```python
from build123d import *

# Parameters (mm, degrees)
BASE_FLANGE1_DEPTH             = 400
SKETCH6_R                      = 2.5
CUT_EXTRUDE2_DEPTH             = 451
SKETCH10_R                     = 6
CUT_EXTRUDE1_DEPTH             = 451
KENAR_FLAN_1_STRIP_CUT_DEPTH   = 192.5268
KENAR_FLAN_1_STRIP_CUT_2_DEPTH = 192.5268
KENAR_FLAN_1_DEPTH             = 192.5268
KENAR_FLAN_1_BEND_DEPTH        = 192.5268


# Sheet-metal steps are written as plain solids
with BuildPart() as part:
    # Sketch1 → Base-Flange1 (new, symmetric)
    with BuildSketch(Plane(origin=(0, 0, 0), x_dir=(0, 0, -1), z_dir=(1, 0, 0))):
        with BuildLine():
            Line((-100, -50), (-100, -3.7366))
            ThreePointArc((-100, -3.7366), (-98.905575199, -1.094424801), (-96.2634, 0))
            Line((-96.2634, 0), (96.2634, 0))
            ThreePointArc((96.2634, 0), (98.905575199, -1.094424801), (100, -3.7366))
            Line((100, -3.7366), (100, -50))
            Line((100, -50), (97, -50))
            Line((97, -50), (97, -3.7366))
            ThreePointArc((97, -3.7366), (96.784254855, -3.215745145), (96.2634, -3))
            Line((96.2634, -3), (-96.2634, -3))
            ThreePointArc((-96.2634, -3), (-96.784254855, -3.215745145), (-97, -3.7366))
            Line((-97, -3.7366), (-97, -50))
            Line((-97, -50), (-100, -50))
        make_face()
    extrude(amount=BASE_FLANGE1_DEPTH, both=True)

    # Sketch6 → Cut-Extrude2 (cut, through all)
    with BuildSketch(Plane(origin=(0, 0, -100), x_dir=(-1, 0, 0), z_dir=(0, 0, -1))):
        with Locations(Location((-385, -15, 0), (0, 0, 90))):
            Circle(SKETCH6_R)
        with Locations(Location((-385, -35, 0), (0, 0, 90))):
            Circle(SKETCH6_R)
    cut_extrude2 = extrude(amount=-CUT_EXTRUDE2_DEPTH, mode=Mode.SUBTRACT)

    # Sketch10 → Cut-Extrude1 (cut, through all)
    with BuildSketch(Plane(origin=(0, 0, -100), x_dir=(-1, 0, 0), z_dir=(0, 0, -1))):
        with Locations(Location((-335, -12.5, 0), (0, 0, 90))):
            Circle(SKETCH10_R)
        with Locations(Location((-335, -37.5, 0), (0, 0, 90))):
            Circle(SKETCH10_R)
    cut_extrude1 = extrude(amount=-CUT_EXTRUDE1_DEPTH, mode=Mode.SUBTRACT)

    # Kenar-Flanş1 strip (across the edge) → Kenar-Flanş1 strip cut (cut)
    with BuildSketch(Plane(origin=(400, -3, -96.2634), x_dir=(-0.42261826174069383, -0.9063077870366526, 0), z_dir=(0, 0, 1))):
        Polygon((-8.343930041, 10.795010968), (-2.649909677, -1.415855108), (0.069013684, -0.148000323), (-5.62500668, 12.062865753), align=None)
    extrude(amount=KENAR_FLAN_1_STRIP_CUT_DEPTH, mode=Mode.SUBTRACT)

    # Kenar-Flanş1 strip 2 (across the edge) → Kenar-Flanş1 strip cut 2 (cut)
    with BuildSketch(Plane(origin=(-400, -3, 96.2634), x_dir=(0.42261826174069383, -0.9063077870366526, 0), z_dir=(0, 0, -1))):
        Polygon((-8.343930041, 10.795010968), (-2.649909677, -1.415855108), (0.069013684, -0.148000323), (-5.62500668, 12.062865753), align=None)
    extrude(amount=KENAR_FLAN_1_STRIP_CUT_2_DEPTH, mode=Mode.SUBTRACT)

    # Kenar-Flanş1 section (across the edge) → Kenar-Flanş1 (add)
    with BuildSketch(Plane(origin=(400, -3, -96.2634), x_dir=(-0.42261826174069383, -0.9063077870366526, 0), z_dir=(0, 0, 1))):
        with BuildLine():
            Line((-3, 0.163300289), (-3, 9.334916012))
            Line((-3, 9.334916012), (0, 9.334916012))
            Line((0, 9.334916012), (0, 0.163300289))
            ThreePointArc((0, 0.163300289), (0.017460361, 0.003870869), (0.069013684, -0.148000323))
            Line((0.069013684, -0.148000323), (-2.649909677, -1.415855108))
            ThreePointArc((-2.649909677, -1.415855108), (-2.91142766, -0.645447973), (-3, 0.163300289))
        make_face()
    extrude(amount=KENAR_FLAN_1_DEPTH)

    # Kenar-Flanş1 section 2 (across the edge) → Kenar-Flanş1 bend (add)
    with BuildSketch(Plane(origin=(-400, -3, 96.2634), x_dir=(0.42261826174069383, -0.9063077870366526, 0), z_dir=(0, 0, -1))):
        with BuildLine():
            Line((-3, 0.163300289), (-3, 9.334916012))
            Line((-3, 9.334916012), (0, 9.334916012))
            Line((0, 9.334916012), (0, 0.163300289))
            ThreePointArc((0, 0.163300289), (0.017460361, 0.003870869), (0.069013684, -0.148000323))
            Line((0.069013684, -0.148000323), (-2.649909677, -1.415855108))
            ThreePointArc((-2.649909677, -1.415855108), (-2.91142766, -0.645447973), (-3, 0.163300289))
        make_face()
    extrude(amount=KENAR_FLAN_1_BEND_DEPTH)

    # Mirror1: Cut-Extrude2, Cut-Extrude1 across plane
    add(cut_extrude2.mirror(Plane(origin=(0, 0, 0), x_dir=(0, 0, 1), z_dir=(1, 0, 0))), mode=Mode.SUBTRACT)
    add(cut_extrude1.mirror(Plane(origin=(0, 0, 0), x_dir=(0, 0, 1), z_dir=(1, 0, 0))), mode=Mode.SUBTRACT)


solid = part.part
```
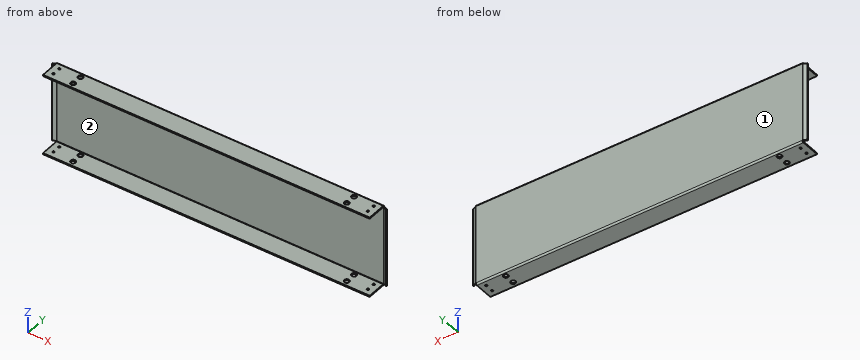
Geometry: final body of the model. Coordinates: model frame, mm. Face numbers are marked on the shaded views. Round coordinates to 2 decimals unless told otherwise and drop trailing zeros. Order: outer loops, then holes, each group sorted by start corner. A loop starts at its lowest first (then second) coordinate and runs counter-clockwise, first axis right, second up. Notation, with made-up numbers: M 84.5,-24.75 L 128.5,-24.75 A22 cw 128.5,-12.75 Z; hole C 85,83 d1. An arc over 180 degrees is marked long. Use one line per item in the form item = value. Start each with the question number.
Q1. Cut plane B-B (x = -146). Return loops of the section in (y, z), and give its area (3 significant figures).
Q2. Cut plane A-A (z = -40.5). Return loops of the section in (x, y), and give its area (3 significant figures).
Q3. Mould query, pull axis X, two halves, no side actions, for the marked faces 1 and 2. Classes: +X half, -X half, draft (parallel to the pull), parting line (faces both ways), or undercut.
Q4. Pin query (flat end, axial travel): pin 1 Ø3 at (y, z) = (-20, -99) entering from -X; pin 2 Ø2 at (x, y) = (-404.5, -2) entering from +Z; pin 3 Ø4.5 at (x, y) = (-385, -35) entering from -Z. Return the tip coordinate at first contact, or that it passes through.
Q5. Material intervals for line 1 (Y direction, x = 335, z = 98); line 2 (Y direction, x = -335, z = -98.1); line 3 (Z direction, x = 155.5, y = -29), sorted ascending. Write a range as [from, to].
Geometry results:
q1.outline = M -50,-100 L -3.74,-100 A3.74 ccw 0,-96.26 L 0,96.26 A3.74 ccw -3.74,100 L -50,100 L -50,97 L -3.74,97 A0.74 cw -3,96.26 L -3,-96.26 A0.74 cw -3.74,-97 L -50,-97 Z
q1.area = 876 mm^2
q2.outline = M -409.73,-4.23 L -408.46,-6.95 L -400.15,-3.07 A0.74 cw -399.84,-3 L 399.84,-3 A0.74 cw 400.15,-3.07 L 408.46,-6.95 L 409.73,-4.23 L 401.42,-0.35 A3.74 ccw 399.84,0 L -399.84,0 A3.74 ccw -401.42,-0.35 Z
q2.area = 2,460 mm^2
q3.face_1 = draft
q3.face_2 = undercut
q4.pin_1 = -400
q4.pin_2 = 96.26
q4.pin_3 = through
q5.line_1 = [-50, -43.5], [-31.5, -18.5], [-6.5, -0.43]
q5.line_2 = [-50, -43.5], [-31.5, -18.5], [-6.5, -0.48]
q5.line_3 = [-100, -97], [97, 100]
